For this review, take the finished solid that the model builds, in its own axes (mm). Face numbers are marked on the shaded views. A direction names the side the tool comes from. Round coordinates to 2 decimals unless told otherwise and drop trailing zeros. Loops run counter-clockwise (first coordinate to the right, second up) from the corner with the lowest first, then second, coordinate; pieces in that order, holes last.
1) Take a section at A-A (y = 0). State the section outline as (x, z) points (3 decimals).
2) Take a section at B-B (x = 0). State the section outline as (y, z) points (3 decimals).
3) Insertion check: pin 1 (5 mm diameter, centred on y = -1, z = 6.5, fed in from -X); pin 2 (5 mm diameter, centred on x = -3, y = -5.5, fed in from -Z); pin 3 (5 mm diameter, centred on x = 2, y = -6.5, fed in from +Z) (3 decimals); pin 4 (1.4 mm diameter, centred on x = -13.5, y = -1, fed in from +Z). Each pin has a flat end and moves straight along its axis. Give the tip position at first contact, or say it passes through.
4) Take a section at D-D (z = 22). State the section outline as (x, y) points.
5) Mouldability with a two-part tool opening along X and no side actions: class the marked faces 1, 2, 3 and 4 as pulls with the +X half, pulls with the -X half, needs draft (parallel to the pull), parting line crosses it, or undercut.
6) Wall thickness on L1, parallel to Y at x = 3, z = 15; L2, parallel to Z at x = 0.5, y = 8.5 (3 decimals); L3, parallel to X at y = 0, z = 18.5: over which ranges is each line inside the solid? List them lowest first.
7) Take a section at C-C (x = 4). State the section outline as (y, z) points (3 decimals).
8) Tool access review of the marked faces 5, 6, 7 and 8: name each direction out of +Z, -Z, +X, -X, +Y, -Y from which nothing blocks a thin tool from reaching the whole face with its end or side.
```python
from build123d import *

# Parameters (mm, degrees)
F0_R     = 12.5
F1_DEPTH = 3.175
F2_W     = 7.63344
F2_H     = 4.692908
F3_DEPTH = 2.286


with BuildPart() as f1:
    # F0 (on Top) → F1 (new body)
    with BuildSketch(Plane.XY):
        Circle(F0_R)
    extrude(amount=F1_DEPTH)

    # F2 (on Front) → F3 (join, symmetric)
    with BuildSketch(Plane.XZ):
        Polygon((-10.613647, 6.779125), (-10.613647, 3.175), (-0.518322, 3.175), (-0.518322, 10.689883), (4.565662, 10.429165), (4.565662, 3.175), (8.606777, 3.175), (8.606777, 10.820241), (6.390681, 17.468527), (6.390681, 27.245419), (10.171079, 24.638249), (13.430044, 24.638249), (11.9961, 27.245419), (10.171079, 30.243667), (4.565662, 31.416893), (4.565662, 35.175), (-4.168362, 35.175), (-4.168362, 31.286534), (-10.613647, 31.286534), (-10.613647, 26.593626), (-2.995135, 26.593626), (-2.995135, 17.33817), (-4.950513, 6.779125), align=None)
        with Locations((-14.430367, 28.94008)):
            Rectangle(F2_W, F2_H)
    extrude(amount=F3_DEPTH, both=True)


solid = f1.part
```
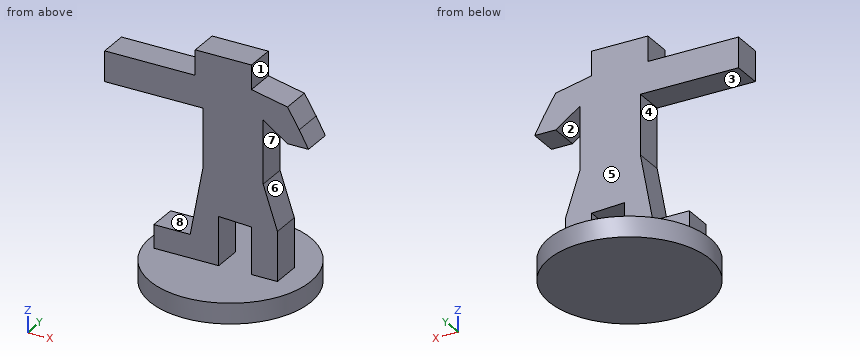
Response:
1. outline: (-18.247, 26.594) - (-2.995, 26.594) - (-2.995, 17.338) - (-4.951, 6.779) - (-10.614, 6.779) - (-10.614, 3.175) - (-12.5, 3.175) - (-12.5, 0) - (12.5, 0) - (12.5, 3.175) - (8.607, 3.175) - (8.607, 10.82) - (6.391, 17.469) - (6.391, 27.245) - (10.171, 24.638) - (13.43, 24.638) - (11.996, 27.245) - (10.171, 30.244) - (4.566, 31.417) - (4.566, 35.175) - (-4.168, 35.175) - (-4.168, 31.287) - (-18.247, 31.287) - close; hole (-0.518, 3.175) - (4.566, 3.175) - (4.566, 10.429) - (-0.518, 10.69) - close
2. outline: (-12.5, 0) - (12.5, 0) - (12.5, 3.175) - (-12.5, 3.175) - close; (-2.286, 10.663) - (2.286, 10.663) - (2.286, 35.175) - (-2.286, 35.175) - close
3. pin 1: stops at x = -10.61
3. pin 2: stops at z = 0
3. pin 3: stops at z = 3.175
3. pin 4: stops at z = 31.29
4. outline: (-3, -2.29) - (6.39, -2.29) - (6.39, 2.29) - (-3, 2.29) - close
5. face 1: pulls with the +X half
5. face 2: undercut
5. face 3: needs draft
5. face 4: pulls with the -X half
6. L1: y = -2.29 to 2.29
6. L2: z = 0 to 3.175
6. L3: x = -3 to 6.39
7. outline: (-11.843, 0) - (11.843, 0) - (11.843, 3.175) - (-11.843, 3.175) - close; (-2.286, 10.458) - (2.286, 10.458) - (2.286, 35.175) - (-2.286, 35.175) - close
8. face 5: +Z, +X, -X, +Y
8. face 6: +X, +Y, -Y
8. face 7: +Y, -Y
8. face 8: -X, +Y, -Y
